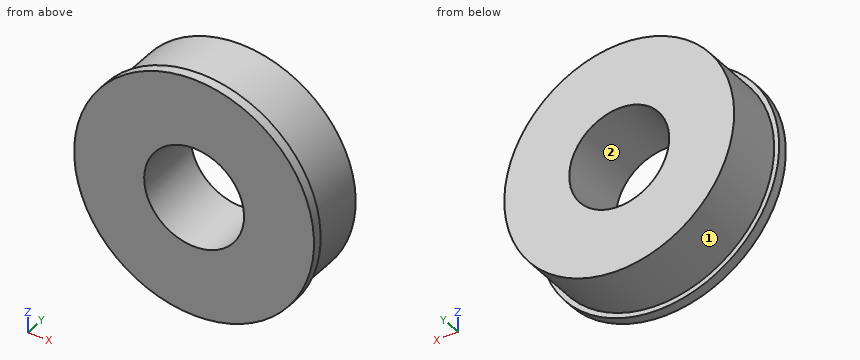
```python
from build123d import *

# Parameters (mm, degrees)
SKETCH1_R           = 12
BOSS_EXTRUDE1_DEPTH = 7
SKETCH2_OUTSIDE_W   = 32.932
SKETCH2_OUTSIDE_H   = 32.932
SKETCH2_OUTSIDE_R   = 11.5
CUT_EXTRUDE3_DEPTH  = 6
CUT_EXTRUDE4_REACH  = 20.358
SKETCH3_R           = 5


with BuildPart() as part:
    # Sketch1 → Boss-Extrude1 (new body)
    with BuildSketch(Plane(origin=(0, 0, 0), x_dir=(1, 0, 0), z_dir=(0, 1, 0))):
        with Locations(Location((0, 0, 0), (0, 0, 270))):
            Circle(SKETCH1_R)
    extrude(amount=BOSS_EXTRUDE1_DEPTH)

    # Sketch2 outside → Cut-Extrude3 (cut)
    with BuildSketch(Plane(origin=(0, 7, 0), x_dir=(1, 0, 0), z_dir=(0, 1, 0))):
        Rectangle(SKETCH2_OUTSIDE_W, SKETCH2_OUTSIDE_H)
        with Locations(Location((0, 0, 0), (0, 0, 270))):
            Circle(SKETCH2_OUTSIDE_R, mode=Mode.SUBTRACT)
    extrude(amount=-CUT_EXTRUDE3_DEPTH, mode=Mode.SUBTRACT)

    # Sketch3 → Cut-Extrude4 (cut, up to next)
    with BuildSketch(Plane(origin=(0, 7, 0), x_dir=(1, 0, 0), z_dir=(0, 1, 0)), mode=Mode.PRIVATE) as cut_extrude4_sk1:
        with Locations(Location((0, 0, 0), (0, 0, 270))):
            Circle(SKETCH3_R)
    cut_extrude4_tool1 = extrude(cut_extrude4_sk1.sketch, amount=-CUT_EXTRUDE4_REACH, mode=Mode.PRIVATE) & part.part
    add(cut_extrude4_tool1.solids().sort_by_distance((0, 7, 0))[0], mode=Mode.SUBTRACT)


solid = part.part
```
Here's how the part is built. I have some questions about the finished solid (model axes, mm). Face numbers are marked on the shaded views. A direction names the side the tool comes from. Give positions to 0.01 mm unless a question says otherwise; leave off trailing zeros. Order: outer loops, then holes, each group sorted by start corner. A loop starts at its lowest first (then second) coordinate and runs counter-clockwise, first axis right, second up. Notation, with made-up numbers: (19.5, 58) -> (62.5, 58) arc R13 ccw to (62.5, 69) -> close; hole circle Ø11 at (61.5, -37.75). An arc over 180 degrees is marked (long way). Use CSV: the item, a comma, the result in double quotes. Start each with the question number.
Item 1: Suppose I cut it at D-D (z = -10). List the corners of the cut face in (x, y) for me.
Item 2: Suppose I cut it at C-C (y = 0.5). List the corners of the cut face in (x, z) for me.
Item 3: On a 3-axis mill with a long thin cutter (end or side, diameter ignored), from which of +Z, -Z, +X, -X, +Y, -Y can I reach the whole of each face in a straight line? I mean the marked faces 1 and 2. Say none if no direction works.
Item 4: If I drill on probe 1 along X at (y, z) = (2.5, 0); probe 2 along X at (y, z) = (0.5, -4.5); probe 3 along Z at (x, y) = (3.25, 6.75), over which ranges is the centre line in solid material (lowest first)? Write a range as [from, to].
Item 5: I'm going to push flat-ended pins straight in: P1, Ø1, axis at x = -6, y = 1, coming from the -Z side; P2, Ø2, axis at x = 3, y = 4.5, coming from the -Z side; P3, Ø1, axis at x = 4, y = 3, coming from the -Z side. Where does each tip first touch, or does it pass through?
Item 6: Suppose I cut it at A-A (x = 0). List the corners of the cut face in (y, z) for me, and give its area (3 significant figures).
Item 7: Suppose I cut it at B-B (z = 0). List the corners of the cut face in (x, y) for me, and give its area (3 significant figures).
Answer block:
1,outline,"(-6.63, 0) -> (6.63, 0) -> (6.63, 1) -> (5.68, 1) -> (5.68, 7) -> (-5.68, 7) -> (-5.68, 1) -> (-6.63, 1) -> close"
2,outline,"circle Ø24 at (0, 0); hole circle Ø10 at (0, 0)"
3,face 1,"+Y"
3,face 2,"+Y, -Y"
4,probe 1,"x = [-11.5, -5], [5, 11.5]"
4,probe 2,"x = [-11.12, -2.18], [2.18, 11.12]"
4,probe 3,"z = [-11.03, -3.8], [3.8, 11.03]"
5,P1,"stops at z = -10.67"
5,P2,"stops at z = -11.32"
5,P3,"stops at z = -10.95"
6,outline,"(0, -12) -> (1, -12) -> (1, -11.5) -> (7, -11.5) -> (7, -5) -> (0, -5) -> close; (0, 5) -> (7, 5) -> (7, 11.5) -> (1, 11.5) -> (1, 12) -> (0, 12) -> close"
6,area,"92.0 mm^2"
7,outline,"(-12, 0) -> (-5, 0) -> (-5, 7) -> (-11.5, 7) -> (-11.5, 1) -> (-12, 1) -> close; (5, 0) -> (12, 0) -> (12, 1) -> (11.5, 1) -> (11.5, 7) -> (5, 7) -> close"
7,area,"92.0 mm^2"
